```python
from build123d import *

# Parameters (mm, degrees)
F0_R            = 10
F0_R_2          = 6.65
F1_DEPTH        = 3
F3_DEPTH        = 3
F3_COPIES_COUNT = 9


# Not quite as in the source:
# - a pattern or mirror of a feature is missing from the dataset's text; its kind, count and spacing are read off the source's solid
# - a feature names something its author has since deleted; it is built from what else it names


with BuildPart() as f1:
    # F0 (on Top) → F1 (new body)
    with BuildSketch(Plane.XY):
        Circle(F0_R)
        Circle(F0_R_2, mode=Mode.SUBTRACT)
    extrude(amount=F1_DEPTH)

    # F2 (on Top) → F3 (join, through all)
    with BuildSketch(Plane.XY):
        with BuildLine():
            ThreePointArc((0, 3.7286332735), (-0.3629275105, 5.527055954), (1.161605891, 6.5477608199))
            ThreePointArc((1.161605891, 6.5477608199), (0, 6.65), (-1.161605891, 6.5477608199))
            ThreePointArc((-1.161605891, 6.5477608199), (-1.6872745189, 4.8988804099), (-1.161605891, 3.25))
            Line((-1.161605891, 3.25), (0, 3.25))
            Line((0, 3.25), (0, 3.7286332735))
        make_face()
    f3 = extrude(amount=F3_DEPTH)

    # F3_copies: F3 ×9 about axis
    f3_copies_axis = Axis((0, 0, 0), (0, 0, 1))
    for i in range(1, F3_COPIES_COUNT):
        add(f3.rotate(f3_copies_axis, i * 360 / F3_COPIES_COUNT))


solid = f1.part
```
CAD build for the part. Positions are in the model's coordinates, mm. Coordinates: 2 decimals unless noted, no trailing zeros. Write each loop counter-clockwise with the first axis right and the second up, starting at its lowest first coordinate (ties: lowest second). Pieces come first, ordered by that corner, then holes.
(1) Flat gauge pins, fed straight in: pin 1 (1.5 mm diameter, centred on y = -1, z = 1.5, fed in from -X); pin 2 (1.5 mm diameter, centred on y = 7.5, z = 2, fed in from -X). Where does each tip first touch, or does it go through?
(2) Drill centre lines: probe 1 along Y at (x, z) = (-2.75, 1.25); probe 2 along Y at (x, z) = (-3.75, 0.9); probe 3 along Y at (x, z) = (-4.25, 2.2). Where is each one in solid material? Low to high.
(3) Two-plate mould, pull along Y, no slides. Class faces 1 (the face through (-0.1, -4.3, 0)), 2 (the face through (3.251, 4.454, 1.479)), 3 (the face through (-2.17, -9.76, 1.48)): +Y half, -Y half, draft (parallel to the pull), parting line (faces both ways), or undercut.
(4) Cut at A-A, the plane y = 8.5. List the corners of the cut face in (x, z), and give its area (3 significant figures).
Geometry says:
1. pin 1: stops at x = -10
1. pin 2: stops at x = -7.38
2. probe 1: y = -9.61 to -5.85, -3.4 to -1.74, 1.94 to 2.93, 6.05 to 9.61
2. probe 2: y = -9.27 to -5.49, -4.08 to -2.7, -0.72 to 0.6, 2.07 to 3.8, 5.2 to 9.27
2. probe 3: y = -9.05 to -5.11, -4.23 to -2.99, -0.83 to 0.39, 2.46 to 9.05
3. face 1: draft
3. face 2: undercut
3. face 3: parting line
4. outline: (-5.27, 0) - (5.27, 0) - (5.27, 3) - (-5.27, 3) - close
4. area: 31.6 mm2
